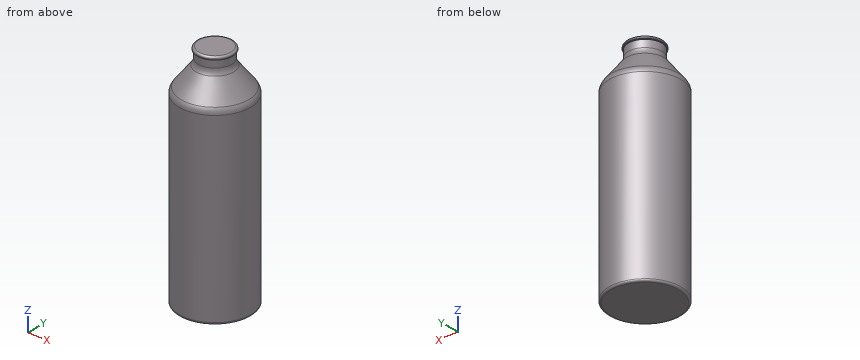
```python
from build123d import *


with BuildPart() as f1:
    # F0 (on Front) → F1 (revolve)
    with BuildSketch(Plane.XZ):
        with BuildLine():
            Line((0, 230), (0, 0))
            Line((0, 0), (34.425, 0))
            ThreePointArc((34.425, 0), (35.839214, 0.585786), (36.425, 2))
            Line((36.425, 2), (36.425, 187.571632))
            ThreePointArc((36.425, 187.571632), (35.884518, 190.814703), (34.321498, 193.70721))
            Line((34.321498, 193.70721), (19.103502, 213.29279))
            ThreePointArc((19.103502, 213.29279), (17.540482, 216.185297), (17, 219.428368))
            Line((17, 219.428368), (17, 226.75))
            ThreePointArc((17, 226.75), (17.073223, 226.926777), (17.25, 227))
            Line((17.25, 227), (17.85, 227))
            ThreePointArc((17.85, 227), (18.026777, 227.073223), (18.1, 227.25))
            Line((18.1, 227.25), (18.1, 228))
            ThreePointArc((18.1, 228), (17.514214, 229.414214), (16.1, 230))
            Line((16.1, 230), (0, 230))
        make_face()
    revolve(axis=Axis((0, 0, 115), (0, 0, 1)))


solid = f1.part
```
Check sheet for the modelled part. Datum: model origin and axes. Units: mm. Coordinates: 2 decimals unless noted, no trailing zeros. Write each loop counter-clockwise with the first axis right and the second up, starting at its lowest first coordinate (ties: lowest second). Pieces come first, ordered by that corner, then holes. Notation, with made-up numbers: M 23,-31 L 79,-31 A20 cw 79,-6 Z; hole C -9.5,18 d8. An arc over 180 degrees is marked long. Write item = value, one per line. Start each with the question number.
1. Sectioned sample at C-C (z = 103). Record the cut outline in (x, y) (3 decimals).
2. Go/stop test with flat-tipped pins: pin 1 (8 mm diameter, centred on x = 24, y = 25.5, fed in from -Z); pin 2 (10 mm diameter, centred on y = -7, z = 167, fed in from -X); pin 3 (4 mm diameter, centred on y = 27.5, z = 133.5, fed in from +X); pin 4 (4 mm diameter, centred on y = -14, z = 91.5, fed in from -X). Record where each tip stops, or that it passes through.
3. Thickness scan on probe 1 along X at (y, z) = (-4, 31); probe 2 along X at (y, z) = (32.5, 44.5); probe 3 along Y at (x, z) = (-23.5, 31.5). Record the ranges inside material, lowest first.
The answers:
q1.outline = C 0,0 d72.85
q2.pin_1 = 0
q2.pin_2 = -36.37
q2.pin_3 = 26.01
q2.pin_4 = -34.39
q3.probe_1 = -36.2 to 36.2
q3.probe_2 = -16.45 to 16.45
q3.probe_3 = -27.83 to 27.83
